Part print with two shaded views. Sizes in mm from the minimum x, y, z corner. Give positions to 0.01 mm unless a question says otherwise; leave off trailing zeros. Write each loop counter-clockwise with the first axis right and the second up, starting at its lowest first coordinate (ties: lowest second). Pieces come first, ordered by that corner, then holes.
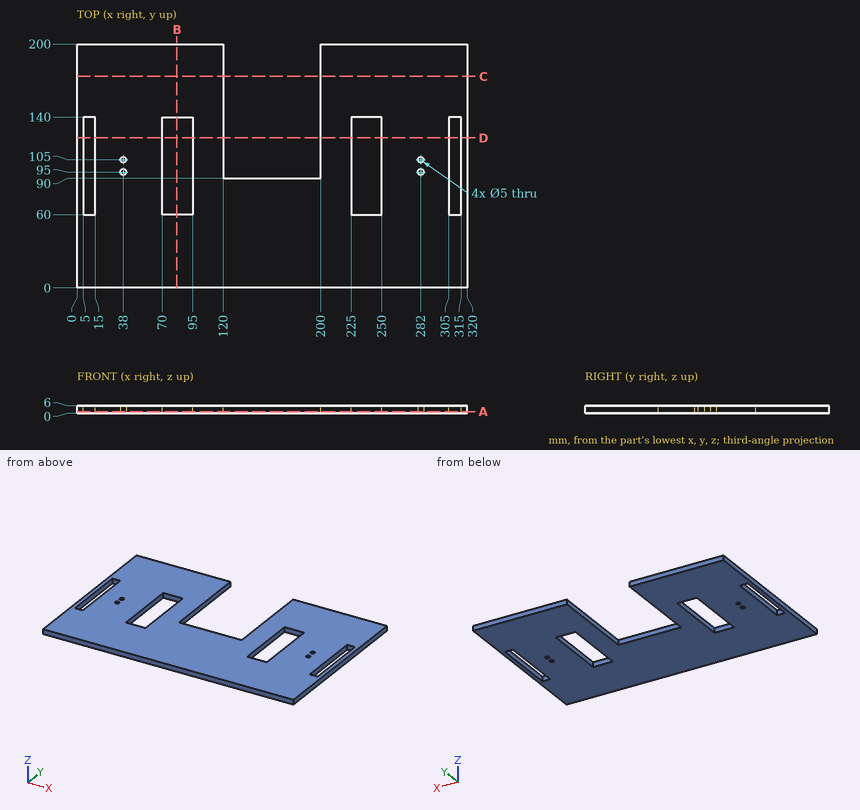
1) Saw through at B-B, the plane x = 82. Write the cut outline in (y, z).
Answers follow:
outline: (0, 0) - (60, 0) - (60, 6) - (0, 6) - close; (140, 0) - (200, 0) - (200, 6) - (140, 6) - close
2) Saw through at A-A, the plane z = 1.2. Count the separate pieces of the cut face and the enclosed holes in it, then the cut area to 3 significant figures.
Answers follow:
separate pieces: 1
enclosed holes: 8
area: 49,500 mm2
3) Pin check, flat tips, straight feed: pin 1 Ø1.5 at (x, z) = (116, 3.5) entering from -Y; pin 2 Ø1.8 at (x, z) = (146.5, 4.5) entering from +Y. Stop position of each tip, or through.
Answers follow:
pin 1: stops at y = 0
pin 2: stops at y = 90
4) Wall check: L1, parallel to X at y = 119.5, z = 5.6; L2, parallel to X at y = 89, z = 2.1; L3, parallel to Y at x = 282, z = 4.3. Give the ranges that are in metal, low to high.
Answers follow:
L1: x = 0 to 5, 15 to 70, 95 to 120, 200 to 225, 250 to 305, 315 to 320
L2: x = 0 to 5, 15 to 70, 95 to 225, 250 to 305, 315 to 320
L3: y = 0 to 92.5, 97.5 to 102.5, 107.5 to 200
5) Saw through at C-C, the plane y = 173.5. Write the cut outline in (x, z), then the cut area to 3 significant figures.
Answers follow:
outline: (0, 0) - (120, 0) - (120, 6) - (0, 6) - close; (200, 0) - (320, 0) - (320, 6) - (200, 6) - close
area: 1,440 mm2
6) Saw through at D-D, the plane y = 123. Write the cut outline in (x, z).
Answers follow:
outline: (0, 0) - (5, 0) - (5, 6) - (0, 6) - close; (15, 0) - (70, 0) - (70, 6) - (15, 6) - close; (95, 0) - (120, 0) - (120, 6) - (95, 6) - close; (200, 0) - (225, 0) - (225, 6) - (200, 6) - close; (250, 0) - (305, 0) - (305, 6) - (250, 6) - close; (315, 0) - (320, 0) - (320, 6) - (315, 6) - close
